Source: CAD feature listing. Evaluate the final solid. Frame: model axes, mm. A direction names the side the tool comes from. Coordinates: 2 decimals unless noted, no trailing zeros. Write each loop counter-clockwise with the first axis right and the second up, starting at its lowest first coordinate (ties: lowest second). Pieces come first, ordered by that corner, then holes. Notation, with made-up numbers: (8, -34.5) - (38, -34.5) arc R8 cw to (38, -30.5) - close; hole circle Ø10 at (78, -33.75). An arc over 180 degrees is marked (long way). One line per item, written item: value.
from build123d import *

# Parameters (mm, degrees)
SKETCH_1_R          = 4.1
SKETCH_1_R_2        = 2.5
EXTRUDE_1_DEPTH     = 10
CUT_EXTRUDE_3_REACH = 92.692
CUT_EXTRUDE_START   = 3
CUT_EXTRUDE_4_DEPTH = 3
SKETCH_7_R          = 5.1
CUT_EXTRUDE_5_DEPTH = 5


with BuildPart() as part:
    # ｽｹｯﾁ1 → ﾎﾞｽ - 押し出し1 (new body)
    with BuildSketch(Plane(origin=(0, 0, 0), x_dir=(1, 0, 0), z_dir=(0, 1, 0))):
        with BuildLine():
            Line((-65, -50), (65, -50))
            ThreePointArc((65, -50), (72.071067812, -47.071067812), (75, -40))
            Line((75, -40), (75, 40))
            ThreePointArc((75, 40), (72.071067812, 47.071067812), (65, 50))
            Line((65, 50), (-65, 50))
            ThreePointArc((-65, 50), (-72.071067812, 47.071067812), (-75, 40))
            Line((-75, 40), (-75, -40))
            ThreePointArc((-75, -40), (-72.071067812, -47.071067812), (-65, -50))
        make_face()
        with Locations(Location((55, 0, 0), (0, 0, 270))):
            Circle(SKETCH_1_R, mode=Mode.SUBTRACT)
        with Locations(Location((43, 12, 0), (0, 0, 270))):
            Circle(SKETCH_1_R_2, mode=Mode.SUBTRACT)
        with Locations(Location((67, 12, 0), (0, 0, 270))):
            Circle(SKETCH_1_R_2, mode=Mode.SUBTRACT)
        with Locations(Location((67, -12, 0), (0, 0, 270))):
            Circle(SKETCH_1_R_2, mode=Mode.SUBTRACT)
        with Locations(Location((43, -12, 0), (0, 0, 270))):
            Circle(SKETCH_1_R_2, mode=Mode.SUBTRACT)
        with Locations(Location((-55, 0, 0), (0, 0, 270))):
            Circle(SKETCH_1_R, mode=Mode.SUBTRACT)
    extrude(amount=EXTRUDE_1_DEPTH)

    # ｽｹｯﾁ5 → ｶｯﾄ - 押し出し3 (cut, up to next)
    with BuildSketch(Plane(origin=(0, 10, 0), x_dir=(1, 0, 0), z_dir=(0, 1, 0)), mode=Mode.PRIVATE) as cut_extrude_3_sk1:
        with BuildLine():
            Line((-20.5, 28.2), (-15.5, 28.2))
            ThreePointArc((-15.5, 28.2), (12.7, 0), (-15.5, -28.2))
            Line((-15.5, -28.2), (-20.5, -28.2))
            ThreePointArc((-20.5, -28.2), (-48.7, 0), (-20.5, 28.2))
        make_face()
    cut_extrude_3_tool1 = extrude(cut_extrude_3_sk1.sketch, amount=-CUT_EXTRUDE_3_REACH, mode=Mode.PRIVATE) & part.part
    # ｽｹｯﾁ5 → ｶｯﾄ - 押し出し3 (cut, up to next)
    with BuildSketch(Plane(origin=(0, 10, 0), x_dir=(1, 0, 0), z_dir=(0, 1, 0)), mode=Mode.PRIVATE) as cut_extrude_3_sk2:
        with BuildLine():
            Line((-20.5, 41.6), (-15.5, 41.6))
            ThreePointArc((-15.5, 41.6), (-13.9, 40), (-15.5, 38.4))
            Line((-15.5, 38.4), (-20.5, 38.4))
            ThreePointArc((-20.5, 38.4), (-22.1, 40), (-20.5, 41.6))
        make_face()
    cut_extrude_3_tool2 = extrude(cut_extrude_3_sk2.sketch, amount=-CUT_EXTRUDE_3_REACH, mode=Mode.PRIVATE) & part.part
    # ｽｹｯﾁ5 → ｶｯﾄ - 押し出し3 (cut, up to next)
    with BuildSketch(Plane(origin=(0, 10, 0), x_dir=(1, 0, 0), z_dir=(0, 1, 0)), mode=Mode.PRIVATE) as cut_extrude_3_sk3:
        with BuildLine():
            Line((-20.5, -38.4), (-15.5, -38.4))
            ThreePointArc((-15.5, -38.4), (-13.9, -40), (-15.5, -41.6))
            Line((-15.5, -41.6), (-20.5, -41.6))
            ThreePointArc((-20.5, -41.6), (-22.1, -40), (-20.5, -38.4))
        make_face()
    cut_extrude_3_tool3 = extrude(cut_extrude_3_sk3.sketch, amount=-CUT_EXTRUDE_3_REACH, mode=Mode.PRIVATE) & part.part
    add(cut_extrude_3_tool1.solids().sort_by_distance((-18, 10, 0))[0], mode=Mode.SUBTRACT)
    add(cut_extrude_3_tool2.solids().sort_by_distance((-18, 10, -40))[0], mode=Mode.SUBTRACT)
    add(cut_extrude_3_tool3.solids().sort_by_distance((-18, 10, 40))[0], mode=Mode.SUBTRACT)

    # ｽｹｯﾁ6 → ｶｯﾄ - 押し出し4 (cut)
    with BuildSketch(Plane(origin=(0, 0, 0), x_dir=(1, 0, 0), z_dir=(0, 1, 0)).offset(CUT_EXTRUDE_START)):
        with BuildLine():
            Line((-20.5, 45.2), (-15.5, 45.2))
            ThreePointArc((-15.5, 45.2), (-11.823044738, 43.676955262), (-10.3, 40))
            Line((-10.3, 40), (-10.3, 27.716421125))
            ThreePointArc((-10.3, 27.716421125), (12.7, 0), (-10.3, -27.716421125))
            Line((-10.3, -27.716421125), (-10.3, -40))
            ThreePointArc((-10.3, -40), (-11.823044738, -43.676955262), (-15.5, -45.2))
            Line((-15.5, -45.2), (-20.5, -45.2))
            ThreePointArc((-20.5, -45.2), (-24.176955262, -43.676955262), (-25.7, -40))
            Line((-25.7, -40), (-25.7, -27.716421125))
            ThreePointArc((-25.7, -27.716421125), (-48.7, 0), (-25.7, 27.716421125))
            Line((-25.7, 27.716421125), (-25.7, 40))
            ThreePointArc((-25.7, 40), (-24.176955262, 43.676955262), (-20.5, 45.2))
        make_face()
    extrude(amount=-CUT_EXTRUDE_4_DEPTH, mode=Mode.SUBTRACT)

    # ｽｹｯﾁ7 → ｶｯﾄ - 押し出し5 (cut)
    with BuildSketch(Plane.XZ):
        with Locations(Location((20, 0, 0), (0, 0, 270))):
            Circle(SKETCH_7_R)
    extrude(amount=-CUT_EXTRUDE_5_DEPTH, mode=Mode.SUBTRACT)


solid = part.part
1) Section query C-C on z = 22.5. Output: boundary loops of the cut face in (x, y).
Values found:
outline: (-75, 0) - (-37.5, 0) - (-37.5, 10) - (-75, 10) - close; (1.5, 0) - (75, 0) - (75, 10) - (1.5, 10) - close
2) Material intervals for line 1 (X direction, y = 2.7, z = 0); line 2 (Z direction, x = -20, y = 5.25); line 3 (Z direction, x = -54.5, y = 6), sorted ascending.
Values found:
line 1: -75 to -59.1, -50.9 to -48.7, 12.7 to 14.9, 25.1 to 50.9, 59.1 to 75
line 2: -50 to -41.6, -38.4 to -28.2, 28.2 to 38.4, 41.6 to 50
line 3: -50 to -4.07, 4.07 to 50
3) Section query B-B on x = 55. Output: boundary loops of the cut face in (y, z).
Values found:
outline: (0, -50) - (10, -50) - (10, -4.1) - (0, -4.1) - close; (0, 4.1) - (10, 4.1) - (10, 50) - (0, 50) - close
4) Section query D-D on x = 20. Output: boundary loops of the cut face in (y, z).
Values found:
outline: (0, -50) - (10, -50) - (10, 50) - (0, 50) - (0, 5.1) - (5, 5.1) - (5, -5.1) - (0, -5.1) - close
5) Draft query along X for faces 4 (the flat face through (16, 10, -1)), 5 (the cylindrical face through (15, 2, 1)), 6 (the cylindrical face through (72.15, 4.93, -46.99)). Return one class per face: released by +X, released by -X, zero draft, split by the parting line, or undercut.
Values found:
face 4: zero draft
face 5: undercut
face 6: released by +X
6) Reachability of faces 1 (the flat face through (-18, 3, 36)), 2 (the cylindrical face through (-13.9, 6.5, -40)), 3 (the cylindrical face through (71.99, 4.93, 47.15)) from +Z, -Z, +X, -X, +Y, -Y: full face, straight path, thin tool, end or side. Return the list, or none.
Values found:
face 1: -Y
face 2: +Y, -Y
face 3: +Z, +X, +Y, -Y
7) Contact query for a flat-ended pin moving along its axis: P1, Ø5, axis at x = 20, z = 0, coming from the -Y side. Output: stop coordinate, or through.
Values found:
P1: y = 5
8) Section query A-A on y = 7.25. State how many separate pieces and enclosed holes the cut face has, then the cut area to 3 significant figures.
Values found:
separate pieces: 1
enclosed holes: 9
area: 11,900 mm2
